Model file for the job. Use its own axes, mm. Face numbers are marked on the shaded views. A direction names the side the tool comes from. Coordinates: 2 decimals unless noted, no trailing zeros. Loops run counter-clockwise (first coordinate to the right, second up) from the corner with the lowest first, then second, coordinate; pieces in that order, holes last. Notation, with made-up numbers: (35.25, -4.75) - (91.25, -4.75) arc R25 ccw to (91.25, 20.25) - close; hole circle Ø6 at (46, 65). An arc over 180 degrees is marked (long way). Write each question's results on one line, items separated by ' | '. Start each with the question number.
```python
from build123d import *

# Parameters (mm, degrees)
SCHIZZO1_W                   = 30
SCHIZZO1_H                   = 5
ESTRUSIONE_ESTRUSIONE1_DEPTH = 10
TAGLIO_ESTRUSIONE1_DEPTH     = 10
SMUSSO1_SIZE                 = 1
SMUSSO2_SIZE                 = 1


with BuildPart() as part:
    # Schizzo1 → Estrusione-Estrusione1 (new body)
    with BuildSketch(Plane.XY):
        with Locations((0, 2.5)):
            Rectangle(SCHIZZO1_W, SCHIZZO1_H)
    extrude(amount=ESTRUSIONE_ESTRUSIONE1_DEPTH)

    # Schizzo2 → Taglio-Estrusione1 (cut)
    with BuildSketch(Plane(origin=(0, 5, 0), x_dir=(1, 0, 0), z_dir=(0, 1, 0))):
        with BuildLine():
            Line((-11, -3.35), (-9, -3.35))
            ThreePointArc((-9, -3.35), (-7.35, -5), (-9, -6.65))
            Line((-9, -6.65), (-11, -6.65))
            ThreePointArc((-11, -6.65), (-12.65, -5), (-11, -3.35))
        make_face()
        with BuildLine():
            Line((11, -3.35), (9, -3.35))
            ThreePointArc((9, -3.35), (7.35, -5), (9, -6.65))
            Line((9, -6.65), (11, -6.65))
            ThreePointArc((11, -6.65), (12.65, -5), (11, -3.35))
        make_face()
    extrude(amount=-TAGLIO_ESTRUSIONE1_DEPTH, mode=Mode.SUBTRACT)

    # Smusso1
    smusso1_edges = [part.edges().sort_by_distance(p)[0] for p in [
        (-15, 2.5, 10),
    ]]
    chamfer(smusso1_edges, length=SMUSSO1_SIZE)

    # Smusso2
    smusso2_edges = [part.edges().sort_by_distance(p)[0] for p in [
        (15, 2.5, 10),
        (15, 2.5, 0),
        (-15, 2.5, 0),
    ]]
    chamfer(smusso2_edges, length=SMUSSO2_SIZE)


solid = part.part
```
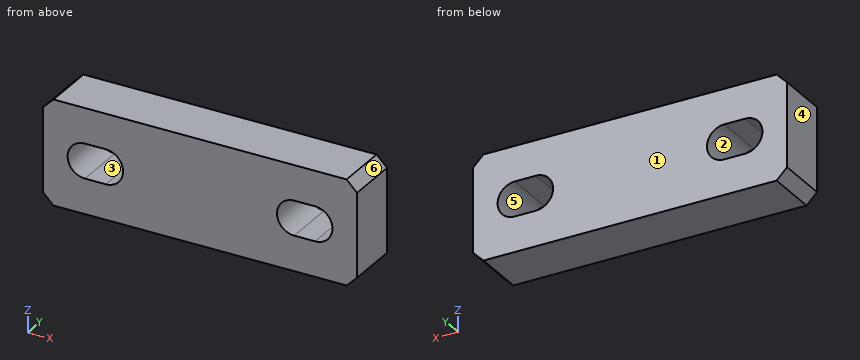
Q1. Which spindle directions (+Z, -Z, +X, -X, +Y, -Y) get a long thin tool onto all of the face, cutting with end or side? Do the marked faces 1 and 2. Say none if no direction does.
Q2. Cut at A-A (x = -10). List the corners of the cut face in (y, z).
Q3. Cut at C-C (z = 6). List the corners of the cut face in (x, y).
Q4. Drill centre lines: L1, parallel to X at y = 3.6, z = 5; L2, parallel to Z at x = 10, y = 1.05; L3, parallel to X at y = 4.5, z = 5.75. Where is each one in solid material? Low to high. Write a range as from..to.
Q5. Mould opens along Z. For the marked faces 3, 4, 5 and 6 say: +Z half, -Z half, draft (parallel to the pull), parting line (faces both ways), or undercut.
Q6. Cut at D-D (z = 0.5). List the corners of the cut face in (x, y), and give its area (3 significant figures).
Q7. Cut at B-B (y = 1.05). List the corners of the cut face in (x, z), and give its area (3 significant figures).
Check result:
1) face 1: +Z, -Z, +X, -X, +Y | face 2: +Y, -Y
2) outline: (0, 0) - (5, 0) - (5, 3.35) - (0, 3.35) - close; (0, 6.65) - (5, 6.65) - (5, 10) - (0, 10) - close
3) outline: (-15, 0) - (-12.31, 0) - (-12.31, 5) - (-15, 5) - close; (-7.69, 0) - (7.69, 0) - (7.69, 5) - (-7.69, 5) - close; (12.31, 0) - (15, 0) - (15, 5) - (12.31, 5) - close
4) L1: -15..-12.65, -7.35..7.35, 12.65..15 | L2: 0..3.35, 6.65..10 | L3: -15..-12.47, -7.53..7.53, 12.47..15
5) face 3: undercut | face 4: draft | face 5: undercut | face 6: +Z half
6) outline: (-14.5, 0) - (14.5, 0) - (14.5, 5) - (-14.5, 5) - close | area: 145 mm²
7) outline: (-15, 1) - (-14, 0) - (14, 0) - (15, 1) - (15, 9) - (14, 10) - (-14, 10) - (-15, 9) - close; hole (-11, 3.35) - (-9, 3.35) arc R1.65 ccw to (-9, 6.65) - (-11, 6.65) arc R1.65 ccw to start; hole (9, 3.35) - (11, 3.35) arc R1.65 ccw to (11, 6.65) - (9, 6.65) arc R1.65 ccw to start | area: 268 mm²
